Build history of the part. All positions in model axes, mm. Face numbers are marked on the shaded views. Coordinates: 2 decimals unless noted, no trailing zeros. Loops run counter-clockwise (first coordinate to the right, second up) from the corner with the lowest first, then second, coordinate; pieces in that order, holes last.
(1) Flat gauge pin, fed straight in: P1, Ø3, axis at x = -7.5, z = -28.54, coming from the +Y side. Where does the tip first touch, or does it go through?
(2) Wall check: L1, parallel to Z at x = -3, y = 3.9; L2, parallel to Z at x = 2.25, y = 1.05; L3, parallel to X at y = 0.9, z = -3. Give the ranges that are in metal, low to high.
(3) Slice it at A-A (x = -7.5). Give the cut face in (y, z), and give its area (4 significant figures).
(4) Slice it at C-C (z = 0). Give the cut face in (x, y).
(5) Slice it at B-B (y = 0.8). Give the cut face in (x, z), and give its area (3 significant figures).
(6) Two-plate mould, pull along X, no slides. Class the marked faces 1, 2 and 3: pulls with the +X half, pulls with the -X half, needs draft (parallel to the pull), parting line crosses it, or undercut.
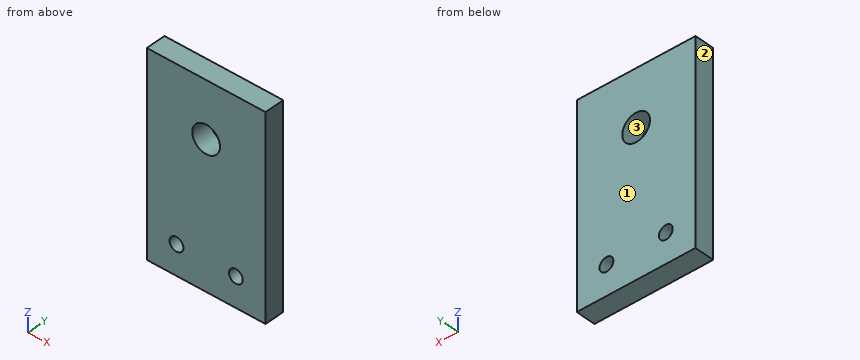
from build123d import *

# Parameters (mm, degrees)
SKETCH_2_W          = 30
SKETCH_2_H          = 50
SKETCH_2_R          = 3.5
EXTRUDE_1_DEPTH     = 5
SKETCH_4_R          = 1.75
CUT_EXTRUDE_1_DEPTH = 10


with BuildPart() as part:
    # 스케치2 → 보스-돌출1 (new body)
    with BuildSketch(Plane(origin=(0, 0, 0), x_dir=(1, 0, 0), z_dir=(0, 1, 0))):
        with Locations((0, 11)):
            Rectangle(SKETCH_2_W, SKETCH_2_H)
        with Locations(Location((0, 0, 0), (0, 0, 270))):
            Circle(SKETCH_2_R, mode=Mode.SUBTRACT)
    extrude(amount=EXTRUDE_1_DEPTH)

    # 스케치4 → 컷-돌출1 (cut)
    with BuildSketch(Plane.XZ):
        with Locations(Location((7.5, -28.539103593, 0), (0, 0, 270))):
            Circle(SKETCH_4_R)
        with Locations(Location((-7.5, -28.539103593, 0), (0, 0, 270))):
            Circle(SKETCH_4_R)
    extrude(amount=-CUT_EXTRUDE_1_DEPTH, mode=Mode.SUBTRACT)


solid = part.part
Response values:
1. P1: passes through
2. L1: z = -36 to -1.8, 1.8 to 14
2. L2: z = -36 to -2.68, 2.68 to 14
2. L3: x = -15 to -1.8, 1.8 to 15
3. outline: (0, -36) - (5, -36) - (5, -30.29) - (0, -30.29) - close; (0, -26.79) - (5, -26.79) - (5, 14) - (0, 14) - close
3. area: 232.5 mm2
4. outline: (-15, 0) - (-3.5, 0) - (-3.5, 5) - (-15, 5) - close; (3.5, 0) - (15, 0) - (15, 5) - (3.5, 5) - close
5. outline: (-15, -36) - (15, -36) - (15, 14) - (-15, 14) - close; hole circle Ø3.5 at (-7.5, -28.54); hole circle Ø7 at (0, 0); hole circle Ø3.5 at (7.5, -28.54)
5. area: 1,440 mm2
6. face 1: needs draft
6. face 2: pulls with the -X half
6. face 3: undercut
